Geometry: final body of the model. Coordinates: model frame, mm. A direction names the side the tool comes from. Round coordinates to 2 decimals unless told otherwise and drop trailing zeros. Write each loop counter-clockwise with the first axis right and the second up, starting at its lowest first coordinate (ties: lowest second). Pieces come first, ordered by that corner, then holes. Notation, with made-up numbers: M 75.25,-18.75 L 111.25,-18.75 A20 cw 111.25,-13.75 Z; hole C 63,42 d6. An arc over 180 degrees is marked long. Put each result on its own line as item: value. Start each with the question number.
```python
from build123d import *

# Parameters (mm, degrees)
BASE_EXTRUDE_DEPTH = 3


with BuildPart() as part:
    # Sketch1 → Base-Extrude (new body)
    with BuildSketch(Plane.XY):
        with BuildLine():
            Line((468.485101771, 336.766175753), (485.987733808, 336.188135391))
            ThreePointArc((485.987733808, 336.188135391), (489.416694784, 338.457661181), (491.026498899, 342.241449149))
            Line((491.026498899, 342.241449149), (492.238136306, 348.965913631))
            Line((492.238136306, 348.965913631), (473.355716317, 349.519727014))
            Line((473.355716317, 349.519727014), (473.445174068, 352.569813696))
            Line((473.445174068, 352.569813696), (485.286157606, 352.222522663))
            ThreePointArc((485.286157606, 352.222522663), (480.454254926, 356.13510234), (476.892234144, 361.230940955))
            Line((476.892234144, 361.230940955), (473.97203133, 360.543616051))
            Line((473.97203133, 360.543616051), (471.7909203, 369.810392981))
            Line((471.7909203, 369.810392981), (474.705571912, 370.496411305))
            Line((474.705571912, 370.496411305), (473.56015142, 375.362901844))
            ThreePointArc((473.56015142, 375.362901844), (470.637669512, 377.921889716), (466.815212769, 378.613369196))
            Line((466.815212769, 378.613369196), (466.789188287, 377.906806581))
            Line((466.789188287, 377.906806581), (466.704790084, 375.615402079))
            Line((466.704790084, 375.615402079), (459.364790084, 375.885752778))
            Line((459.364790084, 375.885752778), (459.475212769, 378.883719894))
            ThreePointArc((459.475212769, 378.883719894), (454.600522802, 379.746395641), (450.113675126, 381.838048014))
            Line((450.113675126, 381.838048014), (448.432649155, 379.353263982))
            Line((448.432649155, 379.353263982), (443.272580982, 382.844194581))
            Line((443.272580982, 382.844194581), (444.953606952, 385.328978613))
            Line((444.953606952, 385.328978613), (433.36986946, 393.165701366))
            Line((433.36986946, 393.165701366), (430.870547605, 394.856562582))
            Line((430.870547605, 394.856562582), (431.68884349, 390.680917334))
            Line((431.68884349, 390.680917334), (435.532374472, 371.067936044))
            ThreePointArc((435.532374472, 371.067936044), (452.26695125, 359.472706568), (461.126484264, 341.142292461))
            ThreePointArc((461.126484264, 341.142292461), (464.265694284, 338.046036211), (468.485101771, 336.766175753))
        make_face()
        Polygon((470.175766233, 343.382194878), (479.67168981, 343.103922683), (479.75956524, 346.102635392), (470.263641663, 346.380907586), align=None, mode=Mode.SUBTRACT)
    extrude(amount=BASE_EXTRUDE_DEPTH)


solid = part.part
```
1) Section C-C, the plane y = 377. Output: boundary loops of the cut face in (x, z), and give its area (3 significant figures).
2) Section D-D, the plane y = 389.5. Output: boundary loops of the cut face in (x, z), and give its area (3 significant figures).
3) Section B-B, the plane z = 1. Output: boundary loops of the cut face in (x, y), and give its area (3 significant figures).
4) Access query for faces 4 (the face through (446, 381, 1)), 5 (the face through (444.1, 384.07, 1.48)), 6 (the face through (489, 338, 1)), 7 (the face through (449.285, 380.613, 1.479)), 8 (the face through (461, 359, 3)). Directions: +Z, -Z, +X, -X, +Y, -Y. A direction counts if a zero-diameter tool reaches every point of the face in a straight line with its end or side. Return the directions, or none.
5) Ray query, probe 1 along X at (y, z) = (389, 1.7); probe 2 along Y at (x, z) = (451.5, 0.85); probe 3 along X at (y, z) = (355.5, 0.7). Return the intervals inside material, ascending.
6) Draft query along X for faces 1 (the face through (475.45, 360.89, 1.48)), 2 (the face through (480.514, 356.071, 1.479)), 3 (the face through (464.21, 338.08, 1.48)). Return one class per face: +X half, -X half, draft (parallel to the pull), parting line (faces both ways), or undercut.
7) First-contact query: pin 1 (1.5 mm diameter, centred on y = 371.5, z = 1.5, fed in from +X). Flat tip, straight axial feed; report the tip coordinate or a pass-through.
8) Section A-A, the plane x = 484.5. Output: boundary loops of the cut face in (y, z), and give its area (3 significant figures).
Solved:
1. outline: M 434.37,0 L 459.41,0 L 459.41,3 L 434.37,3 Z; M 466.76,0 L 472.08,0 L 472.08,3 L 466.76,3 Z
1. area: 91.1 mm2
2. outline: M 431.92,0 L 438.79,0 L 438.79,3 L 431.92,3 Z
2. area: 20.6 mm2
3. outline: M 430.87,394.86 L 435.53,371.07 A40 cw 461.13,341.14 A9.2 ccw 468.49,336.77 L 485.99,336.19 A7.14 ccw 491.03,342.24 L 492.24,348.97 L 473.36,349.52 L 473.45,352.57 L 485.29,352.22 A22.27 cw 476.89,361.23 L 473.97,360.54 L 471.79,369.81 L 474.71,370.5 L 473.56,375.36 A7.28 ccw 466.82,378.61 L 466.7,375.62 L 459.36,375.89 L 459.48,378.88 A19.02 cw 450.11,381.84 L 448.43,379.35 L 443.27,382.84 L 444.95,385.33 Z; hole M 470.18,343.38 L 479.67,343.1 L 479.76,346.1 L 470.26,346.38 Z
3. area: 1,330 mm2
4. face 4: +Z, -Z
4. face 5: +Z, -Z, +X
4. face 6: +Z, -Z, +X, -Y
4. face 7: +Z, -Z, +Y
4. face 8: +Z, +X, -X, +Y, -Y
5. probe 1: x = 432.02 to 439.53
5. probe 2: y = 360.34 to 381.04
5. probe 3: x = 455.26 to 481.07
6. face 1: undercut
6. face 2: +X half
6. face 3: -X half
7. pin 1: stops at x = 474.65
8. outline: M 336.24,0 L 349.19,0 L 349.19,3 L 336.24,3 Z; M 352.25,0 L 352.72,0 L 352.72,3 L 352.25,3 Z
8. area: 40.3 mm2
